Part model, mm, in its own coordinate system. A direction names the side the tool comes from. Give positions to 0.01 mm unless a question says otherwise; leave off trailing zeros. Order: outer loops, then holes, each group sorted by start corner. A loop starts at its lowest first (then second) coordinate and runs counter-clockwise, first axis right, second up. Notation, with made-up numbers: M -24.75,66.25 L -4.75,66.25 A16 cw -4.75,95.25 Z; hole C -37.5,31 d11. An arc over 180 degrees is marked long. Answer as a JSON object with one key per item and string values.
from build123d import *

# Parameters (mm, degrees)
ESQUISSE1_R             = 3.025
ESQUISSE1_R_2           = 0.85
BOSS_EXTRU_1_DEPTH      = 0.75
CONG_2_R                = 1
ESQUISSE2_W             = 12.492816186
ESQUISSE2_H             = 3
ENL_V_MAT_EXTRU_1_DEPTH = 38.373118682
CHANFREIN1_SIZE         = 2
CONG_3_R                = 4
CONG_4_R                = 8


with BuildPart() as part:
    # Esquisse1 → Boss.-Extru.1 (new, symmetric)
    with BuildSketch(Plane.XY):
        with BuildLine():
            Line((-33.5, 16.5), (-19.5, 16.5))
            ThreePointArc((-19.5, 16.5), (-5.589776158, 13.29943825), (5.522918298, 4.34142816))
            ThreePointArc((5.522918298, 4.34142816), (2.059102622, -6.716451548), (-7.007183814, 0.5))
            Line((-7.007183814, 0.5), (-19.5, 0.5))
            Line((-19.5, 0.5), (-33.5, 0.5))
            Line((-33.5, 0.5), (-33.5, 16.5))
        make_face()
        Circle(ESQUISSE1_R, mode=Mode.SUBTRACT)
        with Locations((-30.5, 13.5)):
            Circle(ESQUISSE1_R_2, mode=Mode.SUBTRACT)
        with Locations((-22.5, 13.5)):
            Circle(ESQUISSE1_R_2, mode=Mode.SUBTRACT)
        with Locations((-22.5, 3.5)):
            Circle(ESQUISSE1_R_2, mode=Mode.SUBTRACT)
        with Locations((-30.5, 3.5)):
            Circle(ESQUISSE1_R_2, mode=Mode.SUBTRACT)
    extrude(amount=BOSS_EXTRU_1_DEPTH, both=True)

    # Congé2
    cong_2_edges = [part.edges().sort_by_distance(p)[0] for p in [
        (-33.5, 16.5, 0),
        (-33.5, 0.5, 0),
    ]]
    fillet(cong_2_edges, radius=CONG_2_R)

    # Esquisse2 → Enlèv. mat.-Extru.1 (cut, through all)
    with BuildSketch(Plane.XY.offset(0.75)):
        with Locations((-13.253591907, 2)):
            Rectangle(ESQUISSE2_W, ESQUISSE2_H)
    extrude(amount=-ENL_V_MAT_EXTRU_1_DEPTH, mode=Mode.SUBTRACT)

    # Chanfrein1
    chanfrein1_edges = [part.edges().sort_by_distance(p)[0] for p in [
        (-19.5, 0.5, 0),
    ]]
    chamfer(chanfrein1_edges, length=CHANFREIN1_SIZE)

    # Congé3
    # the kernel refuses this fillet: 4 mm, written as the material it adds along each edge
    with BuildSketch(Plane(origin=(-19.5, 3.5, 0.75), x_dir=(0, -1, 0), z_dir=(0, 0, -1))) as cong_3_piece_1:
        with BuildLine():
            CenterArc((4, -2.645751311), CONG_3_R, 138.590377891, 41.409622109)
            Line((0, -2.645751311), (-0.08, -2.645751311))
            Line((-0.08, -2.645751311), (-0.08, 0))
            Line((-0.08, 0), (0, 0.08))
            ThreePointArc((0, 0.08), (0.5, 0.08), (0.94, 0.052915026))
            Line((0.94, 0.052915026), (1, 0))
        make_face()
    extrude(amount=1.5)

    # Congé4
    cong_4_edges = [part.edges().sort_by_distance(p)[0] for p in [
        (-7.007183814, 3.5, 0),
    ]]
    fillet(cong_4_edges, radius=CONG_4_R)


solid = part.part
1. Pin check, flat tips, straight feed: P1, Ø1.4, axis at x = -30.5, y = 13.5, coming from the +Z side; P2, Ø0.8, axis at x = -28.5, z = 0, coming from the -Y side. Stop position of each tip, or through.
Worked answers:
{"P1": "passes through", "P2": "stops at y = 0.5"}
2. Cut at A-A on x = -22.5. Give the cut face in (y, z).
Worked answers:
{"outline": "M 0.5,-0.75 L 2.65,-0.75 L 2.65,0.75 L 0.5,0.75 Z; M 4.35,-0.75 L 12.65,-0.75 L 12.65,0.75 L 4.35,0.75 Z; M 14.35,-0.75 L 16.5,-0.75 L 16.5,0.75 L 14.35,0.75 Z"}
3. Two-plate mould, pull along Y, no slides. Class faces 4 (the cylindrical face through (-18.287, 3.234, 0.01)), 5 (the cylindrical face through (-23.1, 14.1, 0)), 6 (the cylindrical face through (-31.35, 3.54, -0.01)), 7 (the flat face through (-14, 7, 0.75)): +Y half, -Y half, draft (parallel to the pull), parting line (faces both ways), or undercut.
Worked answers:
{"face 4": "-Y half", "face 5": "undercut", "face 6": "undercut", "face 7": "draft"}
4. Which spindle directions (+Z, -Z, +X, -X, +Y, -Y) get a long thin tool onto all of the face, cutting with end or side? Do faces 1 (the cylindrical face through (-33.199, 16.215, 0.01)), 2 (the flat face through (-27, 0.5, 0)), 3 (the flat face through (-20, 2, 0)). Say none if no direction does.
Worked answers:
{"face 1": "+Z, -Z, -X, +Y", "face 2": "+Z, -Z, -X, -Y", "face 3": "+Z, -Z, -Y"}
5. Cut at B-B on y = 13.5. Give the cut face in (x, z), plus the area to 3 significant figures.
Worked answers:
{"outline": "M -33.5,-0.75 L -31.35,-0.75 L -31.35,0.75 L -33.5,0.75 Z; M -29.65,-0.75 L -23.35,-0.75 L -23.35,0.75 L -29.65,0.75 Z; M -21.65,-0.75 L -6.01,-0.75 L -6.01,0.75 L -21.65,0.75 Z", "area": "36.1 mm^2"}
6. Cut at C-C on x = 2.5. Give the cut face in (y, z), plus the area to 3 significant figures.
Worked answers:
{"outline": "M -6.57,-0.75 L -1.7,-0.75 L -1.7,0.75 L -6.57,0.75 Z; M 1.7,-0.75 L 7.67,-0.75 L 7.67,0.75 L 1.7,0.75 Z", "area": "16.2 mm^2"}
7. Probe line 1 along Y through (x, z) = (-30.5, 0.45); line 2 along X through (y, z) = (1, -0.3); line 3 along X through (y, z) = (1.5, 0.5). List the from-to ranges inside material, lowest first.
Worked answers:
{"line 1": "y = 0.5 to 2.65, 4.35 to 12.65, 14.35 to 16.5", "line 2": "x = -33.37 to -21, -8.53 to -2.85, 2.85 to 6.95", "line 3": "x = -33.5 to -20.5, -9.04 to -2.63, 2.63 to 6.86"}
8. Cut at D-D on z = 0.4. State how many separate pieces and enclosed holes the cut face has, plus the area to 3 significant figures.
Worked answers:
{"separate pieces": "1", "enclosed holes": "5", "area": "553 mm^2"}
